Model file for the job. Use its own axes, mm. A direction names the side the tool comes from. Round coordinates to 2 decimals unless told otherwise and drop trailing zeros. Order: outer loops, then holes, each group sorted by start corner. A loop starts at its lowest first (then second) coordinate and runs counter-clockwise, first axis right, second up. Notation, with made-up numbers: M 34.5,85 L 73.5,85 A5 cw 73.5,91 Z; hole C 48.5,3.5 d5. An arc over 180 degrees is marked long. Return JSON: item names as keys, results as strings. Group by question number.
Item 1: Pin check, flat tips, straight feed: pin 1 Ø9 at (y, z) = (34.5, -38) entering from +X; pin 2 Ø24 at (y, z) = (30, -31.5) entering from -X; pin 3 Ø1.5 at (x, y) = (-113.5, 6.5) entering from -Z. Stop position of each tip, or through.
Item 2: Slice it at B-B on y = 29.5. Write the cut outline in (x, z), then the cut area to 3 significant figures.
Item 3: Slice it at A-A on z = -34.5. Write the cut outline in (x, y).
Item 4: Probe line 1 along Z through (x, y) = (-111, 57.5); line 2 along Z through (x, y) = (-88, 90); line 3 along Z through (x, y) = (-69.5, 5.5). List the from-to ranges inside material, lowest first.
Item 5: Which spindle directions (+Z, -Z, +X, -X, +Y, -Y) get a long thin tool onto all of the face, cutting with end or side? Do faces 1 (the face through (-88.236, 27.641, -36.695)), 2 (the face through (-121.018, 51.018, -84.86)), 3 (the face through (-65.288, 60.106, -36.975)), 4 (the face through (-68.183, 10, -90)). Say none if no direction does.
Item 6: Slice it at D-D on z = -82. Write the cut outline in (x, y), then the cut area to 3 significant figures.
Item 7: Slice it at C-C on x = -73. Write the cut outline in (y, z), then the cut area to 3 significant figures.
Item 8: Pull direction Z, two halves, no side cores. Call faces 5 (the face through (-88.183, 64, -90)), 6 (the face through (-50, 38, -95)), 7 (the face through (-90.905, 14.896, -36.975)): pulls with the +Z half, pulls with the -Z half, needs draft (parallel to the pull), parting line crosses it, or undercut.
from build123d import *

# Parameters (mm, degrees)
SKETCH2_W           = 90
SKETCH2_H           = 120
BOSS_EXTRUDE4_DEPTH = 20
BOSS_EXTRUDE5_DEPTH = 75
SKETCH20_R          = 45
BOSS_EXTRUDE6_DEPTH = 20
SKETCH21_W          = 20
SKETCH21_H          = 100
BOSS_EXTRUDE8_DEPTH = 10
SKETCH26_R          = 5
CUT_EXTRUDE2_DEPTH  = 20
CUT_EXTRUDE3_DEPTH  = 115


with BuildPart() as part:
    # Sketch2 → Boss-Extrude4 (new body)
    with BuildSketch(Plane.XY):
        with Locations((-78.096450442, 37.501466256)):
            Rectangle(SKETCH2_W, SKETCH2_H)
    extrude(amount=BOSS_EXTRUDE4_DEPTH)

    # Sketch19 → Boss-Extrude5 (add)
    with BuildSketch(Plane(origin=(0, 0, 0), x_dir=(-1, 0, 0), z_dir=(0, 0, -1))):
        Polygon((78.096450442, 67.501466256), (52.115688328, 52.501466256), (52.115688328, 22.501466256), (78.096450442, 7.501466256), (104.077212555, 22.501466256), (104.077212555, 52.501466256), align=None)
    extrude(amount=BOSS_EXTRUDE5_DEPTH)

    # Sketch20 → Boss-Extrude6 (add)
    with BuildSketch(Plane(origin=(0, 0, -75), x_dir=(-1, 0, 0), z_dir=(0, 0, -1))):
        with Locations((78.096450442, 37.501466256)):
            Circle(SKETCH20_R)
    extrude(amount=BOSS_EXTRUDE6_DEPTH)


with BuildPart() as body_2:
    # Sketch21 → Boss-Extrude8 (new body)
    with BuildSketch(Plane(origin=(0, 0, -95), x_dir=(-1, 0, 0), z_dir=(0, 0, -1))):
        with Locations((78.183292606, 37.571308656)):
            Rectangle(SKETCH21_W, SKETCH21_H)
    extrude(amount=-BOSS_EXTRUDE8_DEPTH)


with BuildPart() as part_1:
    add(part.part)

    # Combine1: cut body 2
    add(body_2.part, mode=Mode.SUBTRACT)

    # Sketch26 → Cut-Extrude2 (cut)
    with BuildSketch(Plane(origin=(0, 0, -95), x_dir=(-1, 0, 0), z_dir=(0, 0, -1))):
        with Locations((59.346450442, 69.977418898)):
            Circle(SKETCH26_R)
        with Locations((96.846450442, 69.977418898)):
            Circle(SKETCH26_R)
        with Locations((59.346450442, 5.025513614)):
            Circle(SKETCH26_R)
        with Locations((96.846450442, 5.025513614)):
            Circle(SKETCH26_R)
    extrude(amount=-CUT_EXTRUDE2_DEPTH, mode=Mode.SUBTRACT)

    # Sketch28 → Cut-Extrude3 (cut)
    with BuildSketch(Plane.XY.offset(20)):
        Polygon((-58.096450442, 37.501466256), (-78.096450442, 57.501466256), (-98.096450442, 37.501466256), (-78.096450442, 17.501466256), align=None)
    extrude(amount=-CUT_EXTRUDE3_DEPTH, mode=Mode.SUBTRACT)


solid = part_1.part
Output values:
{
 "1": {"pin 1": "x = -52.12", "pin 2": "x = -104.08", "pin 3": "z = 0"},
 "2": {"outline": "M -123.1,0 L -104.08,0 L -104.08,-75 L -122.38,-75 L -122.38,-95 L -90.09,-95 L -90.09,20 L -123.1,20 Z; M -66.1,-95 L -33.81,-95 L -33.81,-75 L -52.12,-75 L -52.12,0 L -33.1,0 L -33.1,20 L -66.1,20 Z", "area": "4,710 mm²"},
 "3": {"outline": "M -104.08,22.5 L -78.1,7.5 L -52.12,22.5 L -52.12,52.5 L -78.1,67.5 L -104.08,52.5 Z; hole M -98.1,37.5 L -78.1,17.5 L -58.1,37.5 L -78.1,57.5 Z"},
 "4": {"line 1": "-95 to -75, 0 to 20", "line 2": "0 to 20", "line 3": "-85 to -75, 0 to 20"},
 "5": {"face 1": "+Z, -Z", "face 2": "-Z", "face 3": "+X, +Y", "face 4": "-Z, +Y, -Y"},
 "6": {"outline": "C -78.1,37.5 d90; hole C -96.85,5.03 d10; hole C -96.85,69.98 d10; hole M -98.1,37.5 L -78.1,17.5 L -58.1,37.5 L -78.1,57.5 Z; hole C -59.35,5.03 d10; hole C -59.35,69.98 d10", "area": "5,250 mm²"},
 "7": {"outline": "M -22.5,0 L 10.44,0 L 10.44,-75 L -7.21,-75 L -7.21,-85 L 22.6,-85 L 22.6,20 L -22.5,20 Z; M 52.41,-85 L 82.21,-85 L 82.21,-75 L 64.56,-75 L 64.56,0 L 97.5,0 L 97.5,20 L 52.41,20 Z", "area": "4,220 mm²"},
 "8": {"face 5": "needs draft", "face 6": "pulls with the -Z half", "face 7": "undercut"}
}
